```python
from build123d import *

# Parameters (mm, degrees)
F1_DEPTH = 19.05
F2_W     = 6.35
F2_H     = 76.2
F3_DEPTH = 12.7
F4_W     = 6.35
F4_H     = 76.2
F5_DEPTH = 12.7


with BuildPart() as f1:
    # F0 (on Right) → F1 (new body)
    with BuildSketch(Plane.YZ):
        Polygon((-279.4, -76.2), (279.4, -76.2), (279.4, -38.1), (292.1, -38.1), (292.1, 38.1), (279.4, 38.1), (279.4, 76.2), (-279.4, 76.2), (-279.4, 38.1), (-292.1, 38.1), (-292.1, -38.1), (-279.4, -38.1), align=None)
    extrude(amount=F1_DEPTH)

    # F2 (on face) → F3 (cut)
    with BuildSketch(Plane.XZ.offset(292.1)):
        with Locations((15.875, 0)):
            Rectangle(F2_W, F2_H)
        with Locations((3.175, 0)):
            Rectangle(F2_W, F2_H)
    extrude(amount=-F3_DEPTH, mode=Mode.SUBTRACT)

    # F4 (on face) → F5 (cut)
    with BuildSketch(Plane(origin=(0, 292.1, 0), x_dir=(-1, 0, 0), z_dir=(0, 1, 0))):
        with Locations((-3.175, 0)):
            Rectangle(F4_W, F4_H)
        with Locations((-15.875, 0)):
            Rectangle(F4_W, F4_H)
    extrude(amount=-F5_DEPTH, mode=Mode.SUBTRACT)


solid = f1.part
```
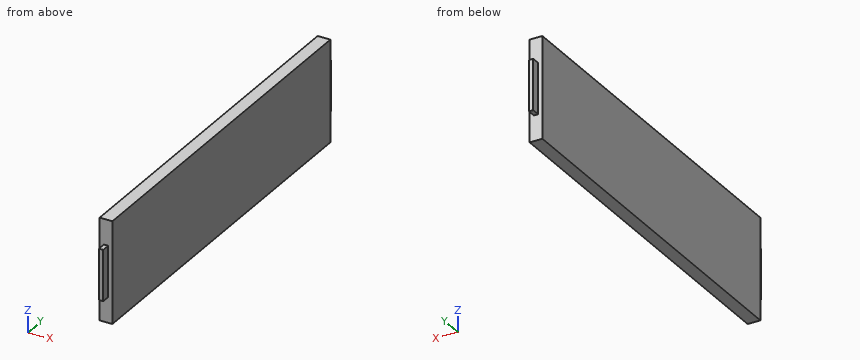
Verification items for the finished model (mm, model axes). Round coordinates to 2 decimals unless told otherwise and drop trailing zeros. Write each loop counter-clockwise with the first axis right and the second up, starting at its lowest first coordinate (ties: lowest second). Pieces come first, ordered by that corner, then holes.
1. Section check B-B on x = 3.25. Enter the section's corners in (y, z), plus the area to 3 significant figures.
2. Gauge pin test, flat ends, axial feed: P1, Ø2, axis at x = 13.5, z = 8, coming from the -Y side; P2, Ø14, axis at y = -287.5, z = -2, coming from the +X side; P3, Ø14, axis at y = -288, z = 4, coming from the -X side; P4, Ø3, axis at x = 9.5, y = 286, coming from the -Z side. Record the tip position at first contact, or that the pin passes through.
3. Scan line: L1, parallel to Y at x = 2.75, z = -21. Record every from-to range of solid material in increasing order.
4. Section check C-C on z = -48. Enter the section's corners in (x, y), plus the area to 3 significant figures.
5. Section check A-A on z = 4.5. Enter the section's corners in (x, y), plus the area to 3 significant figures.
Answer:
1. outline: (-279.4, -76.2) - (279.4, -76.2) - (279.4, 76.2) - (-279.4, 76.2) - close
1. area: 85,200 mm2
2. P1: stops at y = -292.1
2. P2: stops at x = 12.7
2. P3: stops at x = 6.35
2. P4: stops at z = -38.1
3. L1: y = -279.4 to 279.4
4. outline: (0, -279.4) - (19.05, -279.4) - (19.05, 279.4) - (0, 279.4) - close
4. area: 10,600 mm2
5. outline: (0, -279.4) - (6.35, -279.4) - (6.35, -292.1) - (12.7, -292.1) - (12.7, -279.4) - (19.05, -279.4) - (19.05, 279.4) - (12.7, 279.4) - (12.7, 292.1) - (6.35, 292.1) - (6.35, 279.4) - (0, 279.4) - close
5. area: 10,800 mm2
